Check sheet for the drawn part. Datum: minimum x, y, z corner. Units: mm. A direction names the side the tool comes from. Give positions to 0.01 mm unless a question says otherwise; leave off trailing zeros. Order: outer loops, then holes, each group sorted by start corner. A loop starts at its lowest first (then second) coordinate and runs counter-clockwise, first axis right, second up. Notation, with made-up numbers: M 28.5,38.5 L 65.5,38.5 A14 ccw 65.5,47.5 Z; hole C -19,72.25 d5. An arc over 180 degrees is marked long. Put each result on its own line as item: value. Start each with the question number.
Q1. Go/stop test with flat-tipped pins: pin 1 (5 mm diameter, centred on x = 53, y = 34, fed in from +Z) (1 decimal); pin 2 (1 mm diameter, centred on x = 82.5, z = 18.5, fed in from +Y) (1 decimal). Record where each tip stops, or that it passes through.
Q2. Mould release check, pull along X, two halves, no side actions. Record for the marked faces 1, 2, 3 and 4: +X half, -X half, draft (parallel to the pull), parting line (faces both ways), or undercut.
Q3. Section check B-B on y = 44. State how many separate pieces and enclosed holes the cut face has, then the cut area to 3 significant figures.
Q4. Section check A-A on x = 82.55. Record the cut outline in (y, z) (1 decimal), then the cut area to 3 significant figures.
Q5. Access from +Z, -Z, +X, -X, +Y, -Y to the whole of each face (thin tool, end or side, straight path). Record for the marked faces 5 and 6.
Q6. Material ranges on L1, parallel to Y at x = 82, z = 4; L2, parallel to Z at x = 12.7, y = 3.5 (1 decimal); L3, parallel to Y at x = 26, z = 39 (1 decimal), recorded low to high.
Q7. Section check C-C on x = 66.5. Record the cut outline in (y, z) (1 decimal), then the cut area to 3 significant figures.
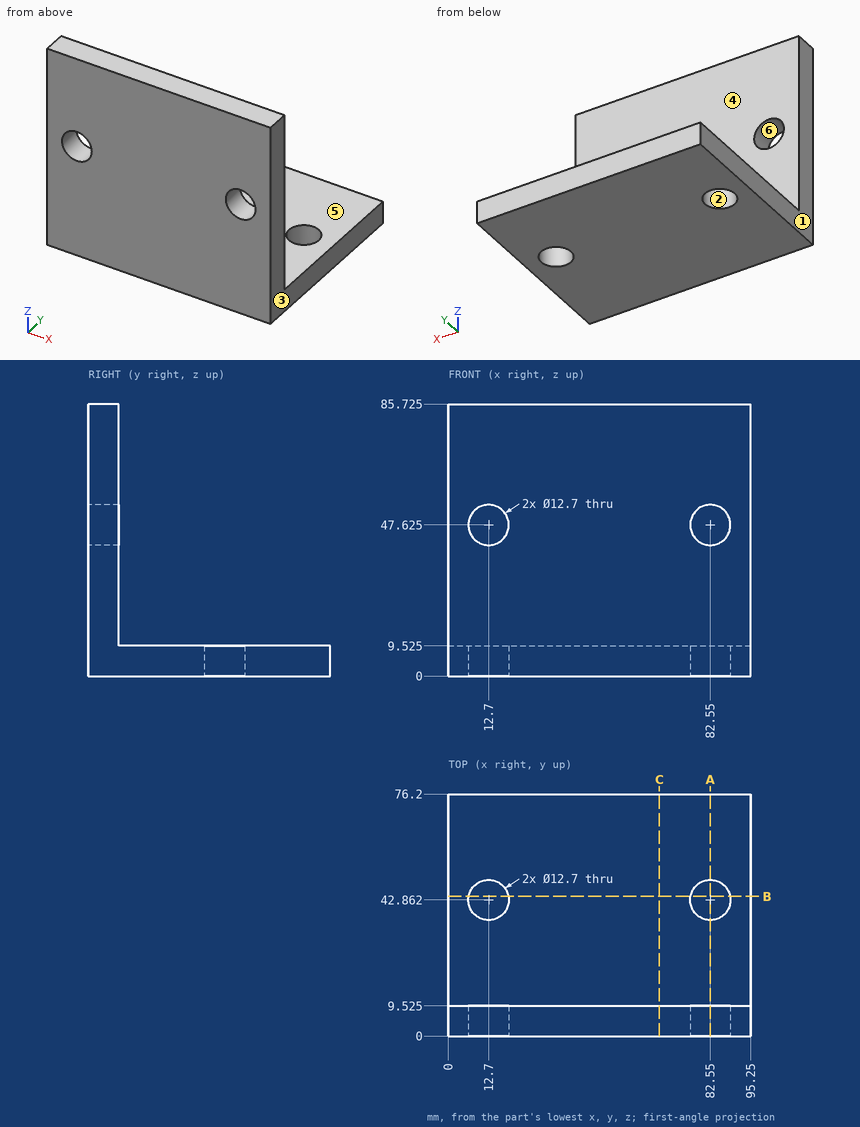
Results found:
1. pin 1: stops at z = 9.5
1. pin 2: stops at y = 9.5
2. face 1: -X half
2. face 2: undercut
2. face 3: +X half
2. face 4: draft
3. separate pieces: 3
3. enclosed holes: 0
3. area: 669 mm^2
4. outline: M 0,0 L 36.5,0 L 36.5,9.5 L 9.5,9.5 L 9.5,41.3 L 0,41.3 Z; M 0,54 L 9.5,54 L 9.5,85.7 L 0,85.7 Z; M 49.2,0 L 76.2,0 L 76.2,9.5 L 49.2,9.5 Z
4. area: 1,210 mm^2
5. face 5: +Z, +X, -X, +Y
5. face 6: +Y, -Y
6. L1: y = 0 to 36.54, 49.19 to 76.2
6. L2: z = 0 to 41.3, 54 to 85.7
6. L3: y = 0 to 9.5
7. outline: M 0,0 L 76.2,0 L 76.2,9.5 L 9.5,9.5 L 9.5,85.7 L 0,85.7 Z
7. area: 1,450 mm^2
